The model under review builds one solid part; all positions refer to its coordinate system, in mm. A direction names the side the tool comes from. Coordinates: 2 decimals unless noted, no trailing zeros. Loops run counter-clockwise (first coordinate to the right, second up) from the corner with the lowest first, then second, coordinate; pieces in that order, holes last. Notation, with made-up numbers: M 50.5,-25 L 65.5,-25 A26 cw 65.5,11 Z; hole C -22.75,82 d8. An arc over 180 degrees is marked long. Return JSON: item names as keys, results as strings.
Autodesk Inventor part; units mm, degrees
ref_plane "YZ Plane" through (0, 0, 0) normal (1, 0, 0) x (0, 1, 0)
ref_plane "XZ Plane" through (0, 0, 0) normal (0, 1, 0) x (-1, 0, 0)
ref_plane "XY Plane" through (0, 0, 0) normal (0, 0, 1) x (1, 0, 0)
sketch "Sketch1" plane through (0, 0, 0) normal (0, 1, 0) x (-1, 0, 0)
  line L0 (-88.9, 127) -> (88.9, 127)
  line L1 (88.9, 127) -> (88.9, -127)
  line L2 (88.9, -127) -> (-88.9, -127)
  line L3 (-88.9, -127) -> (-88.9, 127)
  line L4 (-88.9, 127) -> (88.9, -127) construction
  line L5 (88.9, 127) -> (-88.9, -127) construction
  line L6 (75.9, 114) -> (-75.9, 114)
  line L7 (-75.9, 114) -> (-75.9, -114)
  line L8 (-75.9, -114) -> (75.9, -114)
  line L9 (75.9, -114) -> (75.9, 114)
  point P0 (0, 0)
  dimension "d1" = 254
  dimension "d2" = 177.8
  dimension "d3" = 13
extrude "Extrusion1" add sketch "Sketch1" along normal blind 15.875
shell "Shell1" thickness 2.3622 removed faces 4 at (-75.9, 5.2917, -38) at (25.3, 5.2917, -114) at (75.9, 5.2917, 38) at (-25.3, 5.2917, 114)
hole "Hole1" at (82.25, 15.875, 0) direction (0, -1, 0) diameter 4.496 end up to surface
pattern_linear "Rectangular Pattern1" count 3 spacing 88.9 along (0, 0, 1) of "Hole1" first direction both ways yes
mirror "Mirror1" about plane through (0, 0, 0) normal (1, 0, 0) of "Hole1", "Rectangular Pattern1"
hole "Hole2" at (44.45, 15.875, 120.65) direction (0, -1, 0) diameter 4.496 end up to surface
mirror "Mirror2" about plane through (0, 0, 0) normal (1, 0, 0) of "Hole2"
mirror "Mirror3" about plane through (0, 0, 0) normal (0, 0, 1) of "Hole2", "Mirror2"
properties part number "honeyCombFrame"
1. Add section B-B on x = -50. Give the boundary of the cut face in (y, z) (3 decimals), plus the area to 3 significant figures.
Check values:
{"outline": "M 0,-127 L 15.875,-127 L 15.875,-114 L 13.513,-114 L 13.513,-124.638 L 2.362,-124.638 L 2.362,-114 L 0,-114 Z; M 0,114 L 2.362,114 L 2.362,124.638 L 13.513,124.638 L 13.513,114 L 15.875,114 L 15.875,127 L 0,127 Z", "area": "176 mm²"}
2. Add section C-C on y = 7.75. Give the boundary of the cut face in (x, z).
Check values:
{"outline": "M -88.9,-127 L 88.9,-127 L 88.9,127 L -88.9,127 Z; hole M -86.54,-124.64 L 86.54,-124.64 L 86.54,124.64 L -86.54,124.64 Z"}
3. The part is to be moulded in two halves that separate along Z. For faces 3 (the face through (77, 13.513, 1)), 4 (the face through (-1, 8, -127)), 5 (the face through (-88.9, 8, 2)), say which applies: released by +Z, released by -Z, zero draft, split by the parting line, or undercut.
Check values:
{"face 3": "undercut", "face 4": "released by -Z", "face 5": "zero draft"}
4. Insertion check: pin 1 Ø4 at (x, z) = (-44.45, -120.65) entering from +Y. The pin has a flat end and moves straight along its axis. Give the tip position at first contact, or say it passes through.
Check values:
{"pin 1": "y = 2.36"}
5. To check wall thickness, follow line 1 (X direction, y = 14.15, z = -88.9); line 2 (X direction, y = 14.25, z = -120.65); line 3 (Z direction, x = -44.45, y = 14.1). State the ranges of each line that lie inside material, in increasing order.
Check values:
{"line 1": "-88.9 to -84.5, -80 to -75.9, 75.9 to 80, 84.5 to 88.9", "line 2": "-88.9 to -46.7, -42.2 to 42.2, 46.7 to 88.9", "line 3": "-127 to -122.9, -118.4 to -114, 114 to 118.4, 122.9 to 127"}
6. Add section A-A on z = 69. Give the boundary of the cut face in (x, y) (3 decimals), plus the area to 3 significant figures.
Check values:
{"outline": "M -88.9,0 L -75.9,0 L -75.9,2.362 L -86.538,2.362 L -86.538,13.513 L -75.9,13.513 L -75.9,15.875 L -88.9,15.875 Z; M 75.9,0 L 88.9,0 L 88.9,15.875 L 75.9,15.875 L 75.9,13.513 L 86.538,13.513 L 86.538,2.362 L 75.9,2.362 Z", "area": "176 mm²"}
7. Machinability: for faces 1 (the face through (1, 8, 127)), 2 (the face through (-1, 8, -124.638)), which of the approach directions +Z, -Z, +X, -X, +Y, -Y give a long, thin tool a straight path to every point of the face, cutting with its end or side? Answer none if there is none.
Check values:
{"face 1": "+Z, +X, -X, +Y, -Y", "face 2": "none"}
